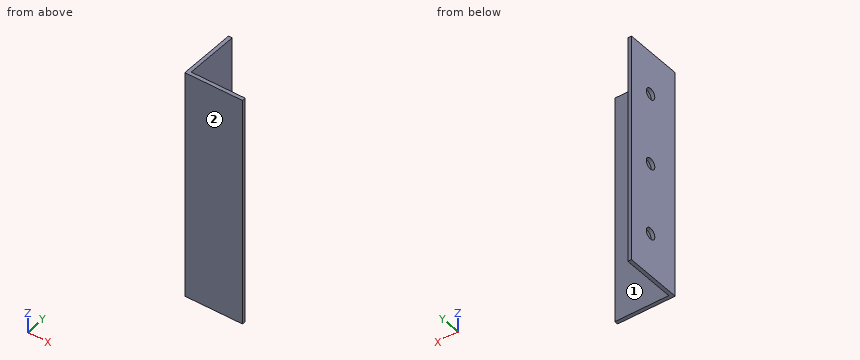
```python
from build123d import *

# Parameters (mm, degrees)
BOSS_EXTRUDE1_DEPTH          = 101.6
F_10_0_1935_DIAMETER_HOLE1_D = 4.9149


with BuildPart() as part:
    # Sketch1 → Boss-Extrude1 (new body)
    with BuildSketch(Plane.XY):
        Polygon((0, 0), (0, 25.4), (1.6002, 25.4), (1.6002, 1.6002), (25.4, 1.6002), (25.4, 0), align=None)
    extrude(amount=BOSS_EXTRUDE1_DEPTH)

    # #10 (0.1935) Diameter Hole1 (through all)
    with Locations(Plane(origin=(1.6002, 0, 0), x_dir=(0, 0, -1), z_dir=(1, 0, 0))):
        with Locations((-82.55, 14.2875), (-50.8, 14.2875), (-19.05, 14.2875)):
            Hole(F_10_0_1935_DIAMETER_HOLE1_D / 2)


solid = part.part
```
The model under review builds one solid part; all positions refer to its coordinate system, in mm. Face numbers are marked on the shaded views. A direction names the side the tool comes from. Give positions to 0.01 mm unless a question says otherwise; leave off trailing zeros. Write each loop counter-clockwise with the first axis right and the second up, starting at its lowest first coordinate (ties: lowest second). Pieces come first, ordered by that corner, then holes.
(1) Consider section B-B, the plane z = 69. Give the boundary of the cut face in (x, y), and give its area (3 significant figures).
(2) To check wall thickness, follow L1, parallel to Y at x = 0.8, z = 82.55; L2, parallel to X at y = 4, z = 61. State the ranges of each line that lie inside material, in increasing order.
(3) Tool access review of the marked faces 1 and 2: name each direction out of +Z, -Z, +X, -X, +Y, -Y from which nothing blocks a thin tool from reaching the whole face with its end or side.
(4) For P1, Ø10, axis at y = 11, z = 17, coming from the -X side; P2, Ø3, axis at x = 18.5, z = 14.5, coming from the +Y side, all flat-tipped, find the tip position at first contact; note any pin that passes through.
(5) Consider section C-C, the plane x = 13.75. Give the boundary of the cut face in (y, z).
(6) Consider section A-A, the plane z = 82.55. Give the boundary of the cut face in (x, y), and give its area (3 significant figures).
Returned:
1. outline: (0, 0) - (25.4, 0) - (25.4, 1.6) - (1.6, 1.6) - (1.6, 25.4) - (0, 25.4) - close
1. area: 78.7 mm2
2. L1: y = 0 to 11.83, 16.74 to 25.4
2. L2: x = 0 to 1.6
3. face 1: +Z, -Z, +X, +Y
3. face 2: +Z, -Z, +X, -X, -Y
4. P1: stops at x = 0
4. P2: stops at y = 1.6
5. outline: (0, 0) - (1.6, 0) - (1.6, 101.6) - (0, 101.6) - close
6. outline: (0, 0) - (25.4, 0) - (25.4, 1.6) - (1.6, 1.6) - (1.6, 11.83) - (0, 11.83) - close; (0, 16.74) - (1.6, 16.74) - (1.6, 25.4) - (0, 25.4) - close
6. area: 70.9 mm2
